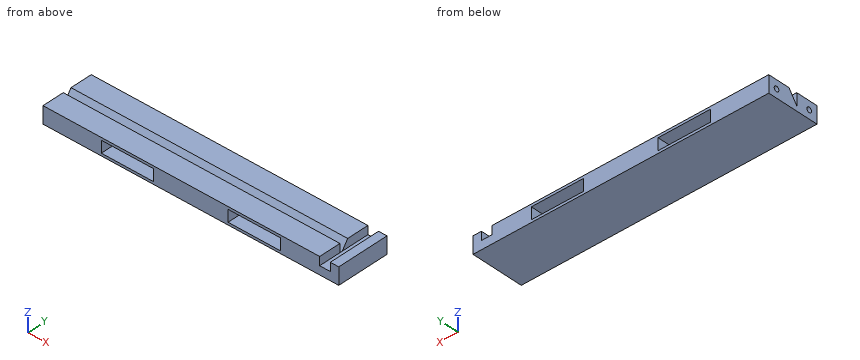
```python
from build123d import *

# Parameters (mm, degrees)
ESBO_O1_W                = 175
ESBO_O1_H                = 31
RESSALTO_EXTRUS_O1_DEPTH = 10
ESBO_O2_W                = 31
ESBO_O2_H                = 7
CORTE_EXTRUS_O1_DEPTH    = 10.5
ESBO_O3_W                = 31
ESBO_O3_H                = 7
CORTE_EXTRUS_O2_DEPTH    = 10.5
ESBO_O5_R                = 1.5
CORTE_EXTRUS_O4_DEPTH    = 8
ESBO_O7_W                = 6.3
ESBO_O7_H                = 31
CORTE_EXTRUS_O6_DEPTH    = 5
CORTE_EXTRUS_O7_DEPTH    = 163.7


with BuildPart() as part:
    # Esboço1 → Ressalto-extrusão1 (new body)
    with BuildSketch(Plane.XY):
        Rectangle(ESBO_O1_W, ESBO_O1_H)
    extrude(amount=RESSALTO_EXTRUS_O1_DEPTH)

    # Esboço2 → Corte-extrusão1 (cut)
    with BuildSketch(Plane(origin=(0, 15.5, 0), x_dir=(1, 0, 0), z_dir=(0, 1, 0))):
        with Locations((-37.5, -5)):
            Rectangle(ESBO_O2_W, ESBO_O2_H)
        with Locations((37.5, -5)):
            Rectangle(ESBO_O2_W, ESBO_O2_H)
    extrude(amount=-CORTE_EXTRUS_O1_DEPTH, mode=Mode.SUBTRACT)

    # Esboço3 → Corte-extrusão2 (cut)
    with BuildSketch(Plane.XZ.offset(15.5)):
        with Locations((-37.5, 5)):
            Rectangle(ESBO_O3_W, ESBO_O3_H)
        with Locations((37.5, 5)):
            Rectangle(ESBO_O3_W, ESBO_O3_H)
    extrude(amount=-CORTE_EXTRUS_O2_DEPTH, mode=Mode.SUBTRACT)

    # Esboço5 → Corte-extrusão4 (cut)
    with BuildSketch(Plane.ZY.offset(87.5)):
        with Locations((5, 10.5)):
            Circle(ESBO_O5_R)
        with Locations((5, -10.5)):
            Circle(ESBO_O5_R)
    extrude(amount=-CORTE_EXTRUS_O4_DEPTH, mode=Mode.SUBTRACT)

    # Esboço7 → Corte-extrusão6 (cut)
    with BuildSketch(Plane.XY.offset(10)):
        with Locations((79.35, 0)):
            Rectangle(ESBO_O7_W, ESBO_O7_H)
    extrude(amount=-CORTE_EXTRUS_O6_DEPTH, mode=Mode.SUBTRACT)

    # Esboço8 → Corte-extrusão7 (cut)
    with BuildSketch(Plane.ZY.offset(87.5)):
        Polygon((10, 2.5), (2.859259966, -2.5), (10, -2.5), align=None)
    extrude(amount=-CORTE_EXTRUS_O7_DEPTH, mode=Mode.SUBTRACT)


solid = part.part
```
Here's how the part is built. I have some questions about the finished solid (model axes, mm). Give positions to 0.01 mm unless a question says otherwise; leave off trailing zeros. Loops run counter-clockwise (first coordinate to the right, second up) from the corner with the lowest first, then second, coordinate; pieces in that order, holes last. Notation, with made-up numbers: (-4.5, 61) -> (14.5, 61) arc R24 ccw to (14.5, 99) -> close; hole circle Ø11 at (45, 11). An arc over 180 degrees is marked (long way). Use one line per item in the form item = value. Start each with the question number.
1) Please list where these lines run through material, in increasing order: line 1 along X through (y, z) = (-9.5, 7); line 2 along X through (y, z) = (-13, 4); line 3 along Y through (x, z) = (-83.75, 5).
2) For P1, Ø1.9, axis at x = 81, y = 2.5, coming from the +Z side; P2, Ø1.5, axis at y = 10, z = 5, coming from the -X side; P3, Ø3.5, axis at x = 40, z = 5.5, coming from the +Y side, each with a flat end and sliding along its axis, tell me the tip position at first contact or that it passes through.
3) Imagine slicing it at A-A (y = -7.5). Please give me the cut outline in (x, z).
4) Imagine slicing it at B-B (x = 48.5). Please give me the cut outline in (y, z).
Check values:
q1.line_1 = -87.5 to -53, -22 to 22, 53 to 76.2, 82.5 to 87.5
q1.line_2 = -87.5 to -53, -22 to 22, 53 to 87.5
q1.line_3 = -15.5 to -12, -9 to -2.5, -1 to 9, 12 to 15.5
q2.P1 = 5
q2.P2 = -79.5
q2.P3 = 5
q3.outline = (-87.5, 0) -> (87.5, 0) -> (87.5, 10) -> (82.5, 10) -> (82.5, 5) -> (76.2, 5) -> (76.2, 10) -> (-87.5, 10) -> close; hole (-53, 1.5) -> (-22, 1.5) -> (-22, 8.5) -> (-53, 8.5) -> close; hole (22, 1.5) -> (53, 1.5) -> (53, 8.5) -> (22, 8.5) -> close
q4.outline = (-15.5, 0) -> (15.5, 0) -> (15.5, 1.5) -> (5, 1.5) -> (5, 8.5) -> (15.5, 8.5) -> (15.5, 10) -> (2.5, 10) -> (-2.5, 2.86) -> (-2.5, 10) -> (-15.5, 10) -> (-15.5, 8.5) -> (-5, 8.5) -> (-5, 1.5) -> (-15.5, 1.5) -> close
